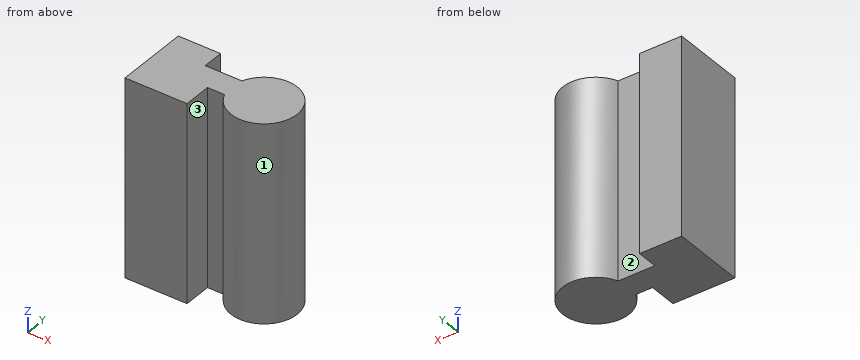
Autodesk Inventor part; units mm, degrees
ref_plane "YZ Plane" through (0, 0, 0) normal (1, 0, 0) x (0, 1, 0)
ref_plane "XZ Plane" through (0, 0, 0) normal (0, 1, 0) x (-1, 0, 0)
ref_plane "XY Plane" through (0, 0, 0) normal (0, 0, 1) x (1, 0, 0)
sketch "Sketch1" plane through (0, 0, 0) normal (0, 0, 1) x (1, 0, 0)
  circle A0 centre (0, 0) radius 2.35
  line L0 (-2.1909, 0.85) -> (-4.8, 0.85)
  line L1 (-4.8, 0.85) -> (-4.8, 2.35)
  line L2 (-2.1909, -0.85) -> (-3.4, -0.85)
  line L3 (-3.4, -0.85) -> (-3.4, -2.85)
  line L4 (-3.4, -2.85) -> (-7.8, -2.85)
  line L5 (-7.8, -2.85) -> (-7.8, 2.35)
  line L6 (-7.8, 2.35) -> (-4.8, 2.35)
  dimension "d0" = 4.7
  dimension "d1" = 4.8
  dimension "d2" = 1.4
  dimension "d3" = 2
  dimension "d7" = 1.7
  dimension "d8" = 3
  dimension "d9" = 2.35
extrude "Extrusion1" add sketch "Sketch1" along normal blind 14
properties part number "rigid connector"
Part model, mm, in its own coordinate system. Face numbers are marked on the shaded views. A direction names the side the tool comes from. Give positions to 0.01 mm unless a question says otherwise; leave off trailing zeros. Loops run counter-clockwise (first coordinate to the right, second up) from the corner with the lowest first, then second, coordinate; pieces in that order, holes last. Notation, with made-up numbers: (61, 69) -> (83, 69) arc R26 ccw to (83, 100) -> close; hole circle Ø2 at (-1, 16). An arc over 180 degrees is marked (long way). Write each question's results on one line, items separated by ' | '. Start each with the question number.
Q1. Which spindle directions (+Z, -Z, +X, -X, +Y, -Y) get a long thin tool onto all of the face, cutting with end or side? Do the marked faces 1, 2 and 3. Say none if no direction does.
Q2. Band-saw the part on B-B on z = 5.5. List the corners of the cut face in (x, y).
Q3. Band-saw the part on C-C on x = 0. List the corners of the cut face in (y, z).
Q4. Pin check, flat tips, straight feed: P1, Ø2, axis at y = -2, z = 10, coming from the +X side; P2, Ø1.6, axis at y = 1.5, z = 7.5, coming from the +X side; P3, Ø3, axis at x = -3, z = 3.5, coming from the +Y side. Stop position of each tip, or through.
Q5. Band-saw the part on A-A on y = 1.4. List the corners of the cut face in (x, z), plus the area to 3 significant figures.
Q6. Wall check: L1, parallel to Y at x = -4.75, z = 9.5; L2, parallel to X at y = -2.4, z = 7; L3, parallel to X at y = -1.55, z = 2. Give the ranges that are in metal, low to high.
Q7. Band-saw the part on D-D on y = -1.15. List the corners of the cut face in (x, z).
Results are:
1) face 1: +Z, -Z | face 2: +Z, -Z, +Y | face 3: +Z, -Z, -Y
2) outline: (-7.8, -2.85) -> (-3.4, -2.85) -> (-3.4, -0.85) -> (-2.19, -0.85) arc R2.35 ccw (long way) to (-2.19, 0.85) -> (-4.8, 0.85) -> (-4.8, 2.35) -> (-7.8, 2.35) -> close
3) outline: (-2.35, 0) -> (2.35, 0) -> (2.35, 14) -> (-2.35, 14) -> close
4) P1: stops at x = 2.13 | P2: stops at x = 2.24 | P3: stops at y = 1.81
5) outline: (-7.8, 0) -> (-4.8, 0) -> (-4.8, 14) -> (-7.8, 14) -> close; (-1.89, 0) -> (1.89, 0) -> (1.89, 14) -> (-1.89, 14) -> close | area: 94.8 mm²
6) L1: y = -2.85 to 0.85 | L2: x = -7.8 to -3.4 | L3: x = -7.8 to -3.4, -1.77 to 1.77
7) outline: (-7.8, 0) -> (-3.4, 0) -> (-3.4, 14) -> (-7.8, 14) -> close; (-2.05, 0) -> (2.05, 0) -> (2.05, 14) -> (-2.05, 14) -> close
